Source: CAD feature listing. Evaluate the final solid. Frame: model axes, mm. A direction names the side the tool comes from. Round coordinates to 2 decimals unless told otherwise and drop trailing zeros. Loops run counter-clockwise (first coordinate to the right, second up) from the corner with the lowest first, then second, coordinate; pieces in that order, holes last. Notation, with made-up numbers: (65.25, 1) -> (122.25, 1) arc R15 cw to (122.25, 21) -> close; hole circle Ø3 at (83, 56.5). An arc over 180 degrees is marked (long way). Return JSON: item names as keys, results as strings. Group by question number.
```python
from build123d import *

# Parameters (mm, degrees)
F0_R          = 15.875
F1_DEPTH      = 6.35
F2_R          = 9.525
F3_DEPTH      = 62.23
F4_SIZE       = 2.54
F5_R          = 2.3876
F6_DEPTH      = 15.876
F6_DEPTH_BACK = 25.4


with BuildPart() as f1:
    # F0 (on Right) → F1 (new body)
    with BuildSketch(Plane.YZ):
        Circle(F0_R)
    extrude(amount=F1_DEPTH)

    # F2 (on face) → F3 (join)
    with BuildSketch(Plane.YZ.offset(6.35)):
        Circle(F2_R)
    extrude(amount=F3_DEPTH)

    # F4
    f4_edges = [f1.edges().sort_by_distance(p)[0] for p in [
        (68.58, -9.525, 0),
    ]]
    chamfer(f4_edges, length=F4_SIZE)

    # F5 (on Front) → F6 (cut, two sides)
    with BuildSketch(Plane.XZ) as f6_sk:
        with Locations((62.23, 0)):
            Circle(F5_R)
    extrude(amount=-F6_DEPTH, mode=Mode.SUBTRACT)
    extrude(f6_sk.sketch, amount=F6_DEPTH_BACK, mode=Mode.SUBTRACT)


solid = f1.part
```
(1) Cut plane C-C (x = 62.23). Return loops of the section in (y, z) (3 decimals).
(2) Ray query, line 1 (X direction, y = -5.5, z = 0); line 2 (X direction, y = 10, z = -3.5); line 3 (Z direction, x = 62, y = 0) (1 decimal). Return the intervals inside material, ascending.
(3) Cut plane B-B (y = 0). Return loops of the section in (x, z) (3 decimals).
(4) Mould query, pull axis Z, two halves, no side actions, for faces 1 (the face through (3.131, -3.441, -15.497)), 2 (the face through (0, 0, 0)), 3 (the face through (59.845, -0.133, 0.105)). Classes: released by +Z, released by -Z, zero draft, split by the parting line, or undercut.
(5) Cut plane A-A (z = 0). Return loops of the section in (x, y) (3 decimals).
(6) Pin query (flat end, axial travel): pin 1 (5 mm diameter, centred on x = 22, y = -10, fed in from +Z); pin 2 (5 mm diameter, centred on x = 25.5, y = -6.5, fed in from -Z); pin 3 (12 mm diameter, centred on y = 10.5, z = -12.5, fed in from -X); pin 4 (6 mm diameter, centred on x = 11, y = 2, fed in from -Z) (3 decimals). Return the tip coordinate at first contact, or that it passes through.
(7) Set-up query: faces 4 (the face through (35.777, 9.085, 2.861)), 5 (the face through (68.58, 0, 0)). Return all of +Z, -Z, +X, -X, +Y, -Y with unobstructed straight access to the full face (end or side cutting, diameter ignored); none if empty.
(8) Cut plane D-D (x = 24). Return loops of the section in (y, z) (3 decimals), and give its area (3 significant figures).
Answers follow:
{
 "1": {"outline": "(-9.221, -2.388) arc R9.525 ccw to (9.221, -2.388) -> close; (-9.221, 2.388) -> (9.221, 2.388) arc R9.525 ccw to start"},
 "2": {"line 1": "0 to 59.84, 64.62 to 68.58", "line 2": "0 to 6.35", "line 3": "-9.5 to -2.4, 2.4 to 9.5"},
 "3": {"outline": "(0, -15.875) -> (6.35, -15.875) -> (6.35, -9.525) -> (66.04, -9.525) -> (68.58, -6.985) -> (68.58, 6.985) -> (66.04, 9.525) -> (6.35, 9.525) -> (6.35, 15.875) -> (0, 15.875) -> close; hole circle Ø4.775 at (62.23, 0)"},
 "4": {"face 1": "split by the parting line", "face 2": "zero draft", "face 3": "undercut"},
 "5": {"outline": "(0, -15.875) -> (6.35, -15.875) -> (6.35, -9.525) -> (59.842, -9.525) -> (59.842, 9.525) -> (6.35, 9.525) -> (6.35, 15.875) -> (0, 15.875) -> close; (64.618, -9.525) -> (66.04, -9.525) -> (68.58, -6.985) -> (68.58, 6.985) -> (66.04, 9.525) -> (64.618, 9.525) -> close"},
 "6": {"pin 1": "z = 5.87", "pin 2": "z = -8.64", "pin 3": "x = 0", "pin 4": "z = -9.525"},
 "7": {"face 4": "+X", "face 5": "+Z, -Z, +X, +Y, -Y"},
 "8": {"outline": "circle Ø19.05 at (0, 0)", "area": "285 mm^2"}
}
